```python
from build123d import *

# Parameters (mm, degrees)
F2_R           = 5.08
F3_DEPTH       = 25.4
F4_R           = 19.62609262
F5_DEPTH       = 21.59
F7_D           = 0.254
F7_DEPTH       = 19.05
F7_CSINK_D     = 19.05
F7_CSINK_ANGLE = 82
F7_TIP         = 0.0763092986


with BuildPart() as f1:
    # F0 (on Front) → F1 (revolve)
    with BuildSketch(Plane.XZ):
        with BuildLine():
            Line((25.2559063932, 69.6122941425), (61.5753642067, 0))
            Line((61.5753642067, 0), (88.9, 0))
            Line((88.9, 0), (88.9, 3.175))
            Line((88.9, 3.175), (67.3492715866, 3.175))
            ThreePointArc((67.3492715866, 3.175), (64.0575636565, 4.0947920019), (61.7194578135, 6.5877058575))
            Line((61.7194578135, 6.5877058575), (28.0708132798, 71.0809412138))
            ThreePointArc((28.0708132798, 71.0809412138), (24.5636545153, 74.8203119971), (19.62609262, 76.2))
            Line((19.62609262, 76.2), (0, 76.2))
            Line((0, 76.2), (0, 73.025))
            Line((0, 73.025), (19.62609262, 73.025))
            ThreePointArc((19.62609262, 73.025), (22.9178005502, 72.1052079981), (25.2559063932, 69.6122941425))
        make_face()
    revolve(axis=Axis((0, 0, 35.2039765567), (0, 0, -1)))

    # F2 (on face) → F3 (cut)
    with BuildSketch(Plane(origin=(0, 0, 0), x_dir=(1, 0, 0), z_dir=(0, 0, -1))):
        with Locations((0, 76.2)):
            Circle(F2_R)
        with Locations((-76.2, 0)):
            Circle(F2_R)
        with Locations((0, -76.2)):
            Circle(F2_R)
        with Locations((76.2, 0)):
            Circle(F2_R)
    extrude(amount=-F3_DEPTH, mode=Mode.SUBTRACT)

    # F4 (on face) → F5 (join)
    with BuildSketch(Plane(origin=(0, 0, 73.025), x_dir=(1, 0, 0), z_dir=(0, 0, -1))):
        Circle(F4_R)
    extrude(amount=F5_DEPTH)

    # F7
    with Locations(Plane(origin=(0, 0, 51.435), x_dir=(1, 0, 0), z_dir=(0, 0, -1))):
        with Locations((0, 0)):
            CounterSinkHole(F7_D / 2, F7_CSINK_D / 2, depth=F7_DEPTH, counter_sink_angle=F7_CSINK_ANGLE)
            with Locations((0, 0, -(F7_DEPTH + F7_TIP / 2))):  # 118° drill point
                Cone(0, F7_D / 2, F7_TIP, mode=Mode.SUBTRACT)


solid = f1.part
```
Model file for the job. Use its own axes, mm. A direction names the side the tool comes from. Coordinates: 2 decimals unless noted, no trailing zeros. Order: outer loops, then holes, each group sorted by start corner. A loop starts at its lowest first (then second) coordinate and runs counter-clockwise, first axis right, second up. Notation, with made-up numbers: (5, 60.5) - (26, 60.5) arc R35 cw to (26, 95.5) - close; hole circle Ø8 at (5, -14.75). An arc over 180 degrees is marked (long way). Return JSON: item names as keys, results as strings. Group by question number.
1) Probe line 1 (Y direction, x = 0, z = 0.7); line 2 (Y direction, x = 0, z = 1); line 3 (Y direction, x = 0.5, z = 62.5). List the from-to ranges inside material, lowest first. Write a range as from..to.
2) Saw through at A-A, the plane x = -76.2. Write the cut outline in (y, z) (1 decimal), plus the area to 3 significant figures.
3) Mould opens along X. For faces 1 (the cylindrical face through (84.795, -26.703, 1.61)), 2 (the cylindrical face through (-0.661, -81.237, 1.565)), 3 (the flat face through (61, 19, 0)) say: released by +X, released by -X, zero draft, split by the parting line, or undercut.
4) Flat gauge pins, fed straight in: P1, Ø1, axis at x = 16.5, z = 49.5, coming from the +Y side; P2, Ø6, axis at y = -13, z = 42.5, coming from the +X side; P3, Ø6, axis at x = -44, y = -54.5, coming from the +Z side; P4, Ø10, axis at x = 54.5, y = 59, coming from the -Z side. Where does each tip first touch, or does it go through?
5) Tool access for faces 4 (the flat face through (-20, -66, 3.175)), 5 (the cylindrical face through (-1.1, 81.16, 1.57)), 6 (the cylindrical face through (10.55, -16.55, 62.38)): list every direction of +Z, -Z, +X, -X, +Y, -Y with a clear straight run to the whole face (end or side of a thin tool).
6) Saw through at C-C, the plane z = 28. Write the cut outline in (x, y).
Values found:
{
 "1": {"line 1": "y = -88.9..-81.28, -71.12..-61.21, 61.21..71.12, 81.28..88.9", "line 2": "y = -88.9..-81.28, -71.12..-61.05, 61.05..71.12, 81.28..88.9", "line 3": "y = -32.54..-28.96, -19.62..19.62, 28.96..32.54"},
 "2": {"outline": "(-45.8, 0) - (-5.1, 0) - (-5.1, 3.2) - (-45.8, 3.2) - close; (5.1, 0) - (45.8, 0) - (45.8, 3.2) - (5.1, 3.2) - close", "area": "259 mm²"},
 "3": {"face 1": "split by the parting line", "face 2": "undercut", "face 3": "zero draft"},
 "4": {"P1": "stops at y = 36.07", "P2": "stops at x = 42.82", "P3": "stops at z = 3.18", "P4": "stops at z = 0"},
 "5": {"face 4": "+Z", "face 5": "+Z, -Z", "face 6": "-Z"},
 "6": {"outline": "circle Ø101.1 at (0, 0); hole circle Ø93.93 at (0, 0)"}
}
